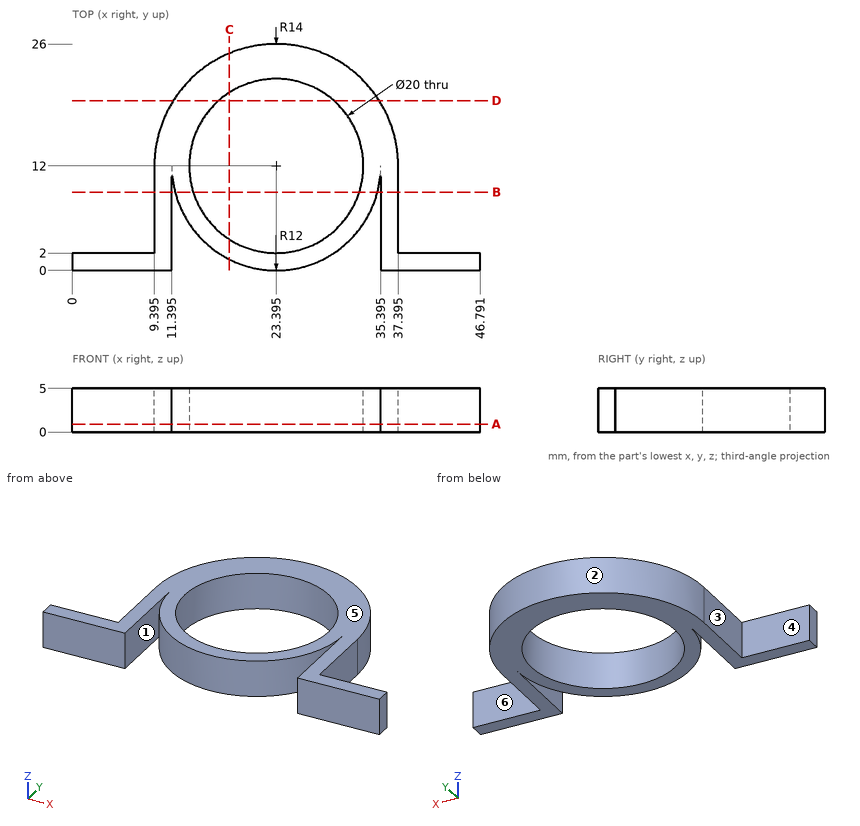
Drawing for the job (mm, zero at the part's lowest x, y, z). A direction names the side the tool comes from. Give positions to 0.01 mm unless a question says otherwise; leave off trailing zeros. Loops run counter-clockwise (first coordinate to the right, second up) from the corner with the lowest first, then second, coordinate; pieces in that order, holes last. Notation, with made-up numbers: M 33,82 L 83,82 A15 cw 83,87 Z; hole C 37,86.5 d10. An arc over 180 degrees is marked long. One line per question, with ' | ' between items. Start each with the question number.
1. Saw through at B-B on y = 9. Give the cut face in (x, z) (1 decimal).
2. Saw through at A-A on z = 0.9. Give the cut face in (x, y) (1 decimal).
3. Saw through at C-C on x = 18. Give the cut face in (y, z).
4. 3-axis set-ups, long thin cutter, end or side, ignore diameter. For the marked faces 4, 5 and 6: which of +Z, -Z, +X, -X, +Y, -Y reach the whole face in a straight line?
5. Flat gauge pins, fed straight in: pin 1 (10 mm diameter, centred on x = 40.5, y = 23, fed in from +Z); pin 2 (1 mm diameter, centred on y = 12, z = 3, fed in from -X) (1 decimal); pin 3 (2 mm diameter, centred on x = 15, z = 1.5, fed in from +Y); pin 4 (1 mm diameter, centred on y = 15, z = 1.5, fed in from -X). Where does each tip first touch, or does it go through?
6. Two-plate mould, pull along X, no slides. Class the marked faces 1, 2 and 3: pulls with the +X half, pulls with the -X half, needs draft (parallel to the pull), parting line crosses it, or undercut.
7. Saw through at D-D on y = 19.5. Give the cut face in (x, z).
8. Probe L1, parallel to X at y = 7.75, z = 3.5 (1 decimal); L2, parallel to Y at x = 21, z = 2.45; L3, parallel to Y at x = 44.5, z = 4. List the from-to ranges inside material, lowest first. Write a range as from..to.
Result sheet:
1) outline: M 9.4,0 L 11.4,0 L 11.4,5 L 9.4,5 Z; M 11.8,0 L 13.9,0 L 13.9,5 L 11.8,5 Z; M 32.9,0 L 35,0 L 35,5 L 32.9,5 Z; M 35.4,0 L 37.4,0 L 37.4,5 L 35.4,5 Z
2) outline: M 0,0 L 11.4,0 L 11.4,12 A12 ccw 35.4,12 L 35.4,0 L 46.8,0 L 46.8,2 L 37.4,2 L 37.4,12 A14 ccw 9.4,12 L 9.4,2 L 0,2 Z; hole C 23.4,12 d20
3) outline: M 1.28,0 L 3.58,0 L 3.58,5 L 1.28,5 Z; M 20.42,0 L 24.92,0 L 24.92,5 L 20.42,5 Z
4) face 4: +Z, -Z, -X, +Y | face 5: +Z, +X, -X, +Y, -Y | face 6: +Z, -Z, +X, +Y
5) pin 1: passes through | pin 2: stops at x = 9.4 | pin 3: stops at y = 23.89 | pin 4: stops at x = 9.62
6) face 1: undercut | face 2: parting line crosses it | face 3: pulls with the -X half
7) outline: M 11.57,0 L 16.78,0 L 16.78,5 L 11.57,5 Z; M 30.01,0 L 35.22,0 L 35.22,5 L 30.01,5 Z
8) L1: x = 9.4..11.4, 12.2..14.3, 32.4..34.6, 35.4..37.4 | L2: y = 0.24..2.29, 21.71..25.79 | L3: y = 0..2
